```python
from build123d import *

# Parameters (mm, degrees)
SKETCH1_W                                      = 95.25
SKETCH1_H                                      = 127
BOSS_EXTRUDE1_DEPTH                            = 12.7
FILLET1_R                                      = 3.175
CBORE_FOR_4_SOCKET_HEAD_CAP_SCREW1_D           = 3.2639
CBORE_FOR_4_SOCKET_HEAD_CAP_SCREW1_CBORE_D     = 5.55752
CBORE_FOR_4_SOCKET_HEAD_CAP_SCREW1_CBORE_DEPTH = 2.8448
SHELL1_START                                   = -9.525
SHELL1_DEPTH                                   = 22.225
SHELL1_START_2                                 = -6.6802
SHELL1_2_DEPTH                                 = 19.3802
CUT_EXTRUDE1_START                             = -2.8448
CUT_EXTRUDE1_DEPTH                             = 2.8448
SKETCH7_W                                      = 40.64
SKETCH7_H                                      = 50.8
BOSS_EXTRUDE2_DEPTH                            = 3.81
F_3_48_TAPPED_HOLE1_D                          = 1.9939
F_3_48_TAPPED_HOLE1_DEPTH                      = 6.35
F_3_48_TAPPED_HOLE1_TIP                        = 0.599027994
FILLET4_R                                      = 6.35
FILLET5_R                                      = 6.35
SKETCH12_R                                     = 6.35
CUT_EXTRUDE2_DEPTH                             = 6.35


# Read off the part's stored shape, not the designer's step: Shell1
with BuildPart() as part:
    # Sketch1 → Boss-Extrude1 (new, symmetric)
    with BuildSketch(Plane(origin=(0, 0, 0), x_dir=(1, 0, 0), z_dir=(0, 1, 0))):
        Rectangle(SKETCH1_W, SKETCH1_H)
    extrude(amount=BOSS_EXTRUDE1_DEPTH, both=True)

    # Fillet1
    fillet1_edges = [part.edges().sort_by_distance(p)[0] for p in [
        (47.625, 0, 63.5),
        (-47.625, 0, 63.5),
        (-47.625, 0, -63.5),
        (47.625, 0, -63.5),
    ]]
    fillet(fillet1_edges, radius=FILLET1_R)

    # CBORE for #4 Socket Head Cap Screw1 (through all)
    with Locations(Plane.XZ.offset(12.7)):
        with Locations((-41.275, -57.15), (-41.275, 57.15), (41.275, 57.15), (41.275, -57.15)):
            CounterBoreHole(CBORE_FOR_4_SOCKET_HEAD_CAP_SCREW1_D / 2, CBORE_FOR_4_SOCKET_HEAD_CAP_SCREW1_CBORE_D / 2, CBORE_FOR_4_SOCKET_HEAD_CAP_SCREW1_CBORE_DEPTH)

    # Shell1 outline → Shell1 (cut)
    with BuildSketch(Plane(origin=(0, 0, 0), x_dir=(1, 0, 0), z_dir=(0, 1, 0)).offset(SHELL1_START)):
        with BuildLine():
            Line((36.238470129, 60.325), (-36.238470129, 60.325))
            ThreePointArc((-36.238470129, 60.325), (-37.06505593, 52.94005593), (-44.45, 52.113470129))
            Line((-44.45, 52.113470129), (-44.45, -52.113470129))
            ThreePointArc((-44.45, -52.113470129), (-37.06505593, -52.94005593), (-36.238470129, -60.325))
            Line((-36.238470129, -60.325), (36.238470129, -60.325))
            ThreePointArc((36.238470129, -60.325), (37.06505593, -52.94005593), (44.45, -52.113470129))
            Line((44.45, -52.113470129), (44.45, 52.113470129))
            ThreePointArc((44.45, 52.113470129), (37.06505593, 52.94005593), (36.238470129, 60.325))
        make_face()
    extrude(amount=SHELL1_DEPTH, mode=Mode.SUBTRACT)

    # Shell1 2 outline → Shell1 2 (cut)
    with BuildSketch(Plane(origin=(0, 0, 0), x_dir=(1, 0, 0), z_dir=(0, 1, 0)).offset(SHELL1_START_2)):
        with BuildLine():
            Line((-36.238470129, 60.325), (-37.665825122, 60.325))
            ThreePointArc((-37.665825122, 60.325), (-37.875973058, 53.750973058), (-44.45, 53.540825122))
            Line((-44.45, 53.540825122), (-44.45, 52.113470129))
            ThreePointArc((-44.45, 52.113470129), (-37.06505593, 52.94005593), (-36.238470129, 60.325))
        make_face()
        with BuildLine():
            Line((37.665825122, 60.325), (36.238470129, 60.325))
            ThreePointArc((36.238470129, 60.325), (37.06505593, 52.94005593), (44.45, 52.113470129))
            Line((44.45, 52.113470129), (44.45, 53.540825122))
            ThreePointArc((44.45, 53.540825122), (37.875973058, 53.750973058), (37.665825122, 60.325))
        make_face()
        with BuildLine():
            ThreePointArc((-36.238470129, -60.325), (-37.06505593, -52.94005593), (-44.45, -52.113470129))
            Line((-44.45, -52.113470129), (-44.45, -53.540825122))
            ThreePointArc((-44.45, -53.540825122), (-37.875973058, -53.750973058), (-37.665825122, -60.325))
            Line((-37.665825122, -60.325), (-36.238470129, -60.325))
        make_face()
        with BuildLine():
            Line((44.45, -53.540825122), (44.45, -52.113470129))
            ThreePointArc((44.45, -52.113470129), (37.06505593, -52.94005593), (36.238470129, -60.325))
            Line((36.238470129, -60.325), (37.665825122, -60.325))
            ThreePointArc((37.665825122, -60.325), (37.875973058, -53.750973058), (44.45, -53.540825122))
        make_face()
    extrude(amount=SHELL1_2_DEPTH, mode=Mode.SUBTRACT)

    # Sketch11 → Cut-Extrude1 (cut)
    with BuildSketch(Plane(origin=(0, -6.6802, 0), x_dir=(1, 0, 0), z_dir=(0, 1, 0)).offset(CUT_EXTRUDE1_START)):
        with BuildLine():
            Line((-44.45, 53.540825122), (-44.45, 52.113470129))
            ThreePointArc((-44.45, 52.113470129), (-37.06505593, 52.94005593), (-36.238470129, 60.325))
            Line((-36.238470129, 60.325), (-37.665825122, 60.325))
            ThreePointArc((-37.665825122, 60.325), (-37.875973058, 53.750973058), (-44.45, 53.540825122))
        make_face()
        with BuildLine():
            Line((44.45, 52.113470129), (44.45, 53.540825122))
            ThreePointArc((44.45, 53.540825122), (37.875973058, 53.750973058), (37.665825122, 60.325))
            Line((37.665825122, 60.325), (36.238470129, 60.325))
            ThreePointArc((36.238470129, 60.325), (37.06505593, 52.94005593), (44.45, 52.113470129))
        make_face()
        with BuildLine():
            Line((-44.45, -52.113470129), (-44.45, -53.540825122))
            ThreePointArc((-44.45, -53.540825122), (-37.875973058, -53.750973058), (-37.665825122, -60.325))
            Line((-37.665825122, -60.325), (-36.238470129, -60.325))
            ThreePointArc((-36.238470129, -60.325), (-37.06505593, -52.94005593), (-44.45, -52.113470129))
        make_face()
        with BuildLine():
            Line((36.238470129, -60.325), (37.665825122, -60.325))
            ThreePointArc((37.665825122, -60.325), (37.875973058, -53.750973058), (44.45, -53.540825122))
            Line((44.45, -53.540825122), (44.45, -52.113470129))
            ThreePointArc((44.45, -52.113470129), (37.06505593, -52.94005593), (36.238470129, -60.325))
        make_face()
    extrude(amount=CUT_EXTRUDE1_DEPTH, mode=Mode.SUBTRACT)

    # Sketch7 → Boss-Extrude2 (add)
    with BuildSketch(Plane(origin=(0, -9.525, 0), x_dir=(1, 0, 0), z_dir=(0, 1, 0))):
        with Locations((-24.13, 0)):
            Rectangle(SKETCH7_W, SKETCH7_H)
    extrude(amount=BOSS_EXTRUDE2_DEPTH)

    # #3-48 Tapped Hole1
    with Locations(Plane(origin=(0, -5.715, 0), x_dir=(-1, 0, 0), z_dir=(0, 1, 0))):
        with Locations((40.767, 0), (7.493, 0)):
            Hole(F_3_48_TAPPED_HOLE1_D / 2, depth=F_3_48_TAPPED_HOLE1_DEPTH)
            with Locations((0, 0, -(F_3_48_TAPPED_HOLE1_DEPTH + F_3_48_TAPPED_HOLE1_TIP / 2))):  # 118° drill point
                Cone(0, F_3_48_TAPPED_HOLE1_D / 2, F_3_48_TAPPED_HOLE1_TIP, mode=Mode.SUBTRACT)

    # Fillet4
    fillet4_edges = [part.edges().sort_by_distance(p)[0] for p in [
        (-3.81, -7.62, 25.4),
        (-3.81, -7.62, -25.4),
        (-44.45, -7.62, -25.4),
        (-44.45, -7.62, 25.4),
    ]]
    fillet(fillet4_edges, radius=FILLET4_R)

    # Fillet5
    fillet5_edges = [part.edges().sort_by_distance(p)[0] for p in [
        (37.665825122, 3.0099, -60.325),
        (44.45, 3.0099, 53.540825122),
        (-44.45, 3.0099, -53.540825122),
        (-37.665825122, 3.0099, 60.325),
        (44.45, 3.0099, -53.540825122),
        (37.665825122, 3.0099, 60.325),
        (-44.45, 3.0099, 53.540825122),
        (-37.665825122, 3.0099, -60.325),
    ]]
    fillet(fillet5_edges, radius=FILLET5_R)

    # Sketch12 → Cut-Extrude2 (cut)
    with BuildSketch(Plane(origin=(0, 0, -63.5), x_dir=(-1, 0, 0), z_dir=(0, 0, -1))):
        with Locations((-21.971, 0.762)):
            Circle(SKETCH12_R)
    extrude(amount=-CUT_EXTRUDE2_DEPTH, mode=Mode.SUBTRACT)


solid = part.part
```
Can you work these out from the model? Positions are in its coordinate system, mm. A direction names the side the tool comes from. Round coordinates to 2 decimals unless told otherwise and drop trailing zeros. Loops run counter-clockwise (first coordinate to the right, second up) from the corner with the lowest first, then second, coordinate; pieces in that order, holes last. Notation, with made-up numbers: (33, 71) -> (69, 71) arc R26 ccw to (69, 92) -> close; hole circle Ø10 at (-13, 39.5). An arc over 180 degrees is marked (long way). Answer in a Markdown table with one row per item.
Item 1: Suppose I cut it at C-C, the plane z = 44. List the corners of the cut face in (x, y) for me (3 decimals).
Answer block:
| item | result |
|---|---|
| outline | (-47.625, -12.7) -> (47.625, -12.7) -> (47.625, 12.7) -> (44.45, 12.7) -> (44.45, -9.525) -> (-44.45, -9.525) -> (-44.45, 12.7) -> (-47.625, 12.7) -> close |
Item 2: Suppose I cut it at A-A, the plane y = -1.25. Give the number of separate pieces and of enclosed holes in the cut face, plus the area to 3 significant figures.
Answer block:
| item | result |
|---|---|
| separate pieces | 1 |
| enclosed holes | 4 |
| area | 1,580 mm² |
Item 3: On a 3-axis mill with a long thin cutter (end or side, diameter ignored), from which of +Z, -Z, +X, -X, +Y, -Y can I reach the whole of each face in a straight line? I mean faces 5 (the cylindrical face through (-46.72, 0.178, 62.545)), 6 (the flat face through (41, -9.855, -59)), 7 (the flat face through (-1, 0, 63.5)), 8 (the flat face through (0, 1, -60.325)), 9 (the cylindrical face through (27.01, -3.1, -61.93)). Say none if no direction works.
Answer block:
| item | result |
|---|---|
| face 5 | +Z, -X, +Y, -Y |
| face 6 | -Y |
| face 7 | +Z, +X, -X, +Y, -Y |
| face 8 | +Y |
| face 9 | -Z |
Item 4: If I drill on probe 1 along X at (y, z) = (-9.25, 0) (3 decimals); probe 2 along X at (y, z) = (0.75, -26.5) (3 decimals); probe 3 along X at (y, z) = (-9.75, 0) (3 decimals), over which ranges is the centre line in solid material (lowest first)?
Answer block:
| item | result |
|---|---|
| probe 1 | -47.625 to -41.764, -39.77 to -8.49, -6.496 to -3.81, 44.45 to 47.625 |
| probe 2 | -47.625 to -44.45, 44.45 to 47.625 |
| probe 3 | -47.625 to -41.764, -39.77 to -8.49, -6.496 to 47.625 |
Item 5: Suppose I cut it at D-D, the plane z = 57.15. List the corners of the cut face in (x, y) for me (3 decimals), plus the area to 3 significant figures.
Answer block:
| item | result |
|---|---|
| outline | (-47.625, -12.7) -> (-44.054, -12.7) -> (-44.054, -9.855) -> (-42.907, -9.855) -> (-42.907, 12.7) -> (-47.625, 12.7) -> close; (-39.643, -9.855) -> (-38.496, -9.855) -> (-38.496, -12.7) -> (38.496, -12.7) -> (38.496, -9.855) -> (39.643, -9.855) -> (39.643, 12.7) -> (36.079, 12.7) -> (36.079, -9.525) -> (-36.079, -9.525) -> (-36.079, 12.7) -> (-39.643, 12.7) -> close; (42.907, -9.855) -> (44.054, -9.855) -> (44.054, -12.7) -> (47.625, -12.7) -> (47.625, 12.7) -> (42.907, 12.7) -> close |
| area | 637 mm² |
Item 6: Suppose I cut it at B-B, the plane x = 13. List the corners of the cut face in (y, z) for me (3 decimals), plus the area to 3 significant figures.
Answer block:
| item | result |
|---|---|
| outline | (-12.7, -63.5) -> (12.7, -63.5) -> (12.7, -60.325) -> (-9.525, -60.325) -> (-9.525, 60.325) -> (12.7, 60.325) -> (12.7, 63.5) -> (-12.7, 63.5) -> close |
| area | 544 mm² |
Item 7: We'd pull the mould along X, two halves only. Please class faces 1 (the flat face through (-47.625, 0, 1)), 2 (the cylindrical face through (-34.42, 1.74, 59.03)), 3 (the flat face through (-24, -5.715, 0)), 4 (the flat face through (-46, 12.7, 0)): released by +X, released by -X, zero draft, split by the parting line, or undercut.
Answer block:
| item | result |
|---|---|
| face 1 | released by -X |
| face 2 | undercut |
| face 3 | undercut |
| face 4 | zero draft |
Item 8: Will these pins go through, and if not, where does the flat tip stop? P1, Ø4.5, axis at x = -41, z = 57.5, coming from the -Y side; P2, Ø2.5, axis at x = -7.493, z = 0, coming from the +Y side (3 decimals).
Answer block:
| item | result |
|---|---|
| P1 | y = -9.86 |
| P2 | y = -5.715 |
